Input: part model. Units: mm. Frame: model coordinates. A direction names the side the tool comes from. Give positions to 0.01 mm unless a question says otherwise; leave off trailing zeros. Write each loop counter-clockwise with the first axis right and the second up, starting at its lowest first coordinate (ties: lowest second). Pieces come first, ordered by that corner, then holes. Notation, with made-up numbers: (1, 82) -> (23, 82) arc R22 cw to (23, 116) -> close; hole circle Ø3 at (-3.5, 35.5). An arc over 180 degrees is marked (long way). Answer as a JSON object with one key per item and string values. Group by question number.
from build123d import *

# Parameters (mm, degrees)
F1_DEPTH = 10
F3_DEPTH = 3
F4_DEPTH = 6


with BuildPart() as f1:
    # F0 (on Right) → F1 (new body)
    with BuildSketch(Plane.YZ):
        Polygon((0, 9), (0, 0), (3, 0), (4, 2), (4.5, 2), (5, 2), (6, 0), (9, 0), (9, 9), align=None)
    extrude(amount=F1_DEPTH)

    # F2 (on face) → F3 (cut)
    with BuildSketch(Plane.XZ):
        Polygon((5, 9), (0, 9), (5, 7.5), align=None)
        Polygon((5, 9), (5, 7.5), (10, 6), (10, 9), align=None)
    extrude(amount=-F3_DEPTH, mode=Mode.SUBTRACT)

    # F2 (on face) → F4 (cut)
    with BuildSketch(Plane.XZ):
        Polygon((5, 9), (5, 7.5), (10, 6), (10, 9), align=None)
    extrude(amount=-F4_DEPTH, mode=Mode.SUBTRACT)


solid = f1.part
1. Section A-A (x = 2). Return the cut outline in (y, z), plus the area to 3 significant figures.
2. Line query: line 1 (Y direction, x = 7, z = 0.75) (3 decimals); line 2 (Z direction, x = 2, y = 4.75); line 3 (Y direction, x = 9, z = 1). Output: solid intervals per line, ascending.
3. Reachability of faces 1 (the face through (4.9, 3.5, 1)), 2 (the face through (7, 6, 8)), 3 (the face through (0, 4, 5)) from +Z, -Z, +X, -X, +Y, -Y: full face, straight path, thin tool, end or side. Return the list, or none.
4. Section D-D (z = 8.5). Return the cut outline in (x, y), plus the area to 3 significant figures.
5. Mould query, pull axis Y, two halves, no side actions, for faces 4 (the face through (5, 0, 4)), 5 (the face through (4.9, 5.5, 1)), 6 (the face through (6, 2.3, 7.2)). Classes: pulls with the +Y half, pulls with the -Y half, needs draft (parallel to the pull), parting line crosses it, or undercut.
6. Contact query for flat-ended pins moving along their axis: pin 1 Ø3 at (y, z) = (8, 5) entering from -X; pin 2 Ø1.6 at (y, z) = (4.5, 8.5) entering from +X. Output: stop coordinate, or through.
7. Section B-B (z = 1.25). Return the cut outline in (x, y) (3 decimals).
8. Section C-C (y = 3.75). Return the cut outline in (x, z), plus the area to 4 significant figures.
Working result:
{
 "1": {"outline": "(0, 0) -> (3, 0) -> (4, 2) -> (5, 2) -> (6, 0) -> (9, 0) -> (9, 9) -> (3, 9) -> (3, 8.4) -> (0, 8.4) -> close", "area": "75.2 mm^2"},
 "2": {"line 1": "y = 0 to 3.375, 5.625 to 9", "line 2": "z = 2 to 9", "line 3": "y = 0 to 3.5, 5.5 to 9"},
 "3": {"face 1": "-Z, +X, -X", "face 2": "+Z, +X, -Y", "face 3": "+Z, -Z, -X, +Y, -Y"},
 "4": {"outline": "(0, 0) -> (1.67, 0) -> (1.67, 3) -> (5, 3) -> (5, 6) -> (10, 6) -> (10, 9) -> (0, 9) -> close", "area": "50.0 mm^2"},
 "5": {"face 4": "pulls with the -Y half", "face 5": "undercut", "face 6": "needs draft"},
 "6": {"pin 1": "stops at x = 0", "pin 2": "stops at x = 5"},
 "7": {"outline": "(0, 0) -> (10, 0) -> (10, 3.625) -> (0, 3.625) -> close; (0, 5.375) -> (10, 5.375) -> (10, 9) -> (0, 9) -> close"},
 "8": {"outline": "(0, 1.5) -> (10, 1.5) -> (10, 6) -> (5, 7.5) -> (5, 9) -> (0, 9) -> close", "area": "63.75 mm^2"}
}
